Could you check a few things on this model? Use its own coordinates, in mm. Face numbers are marked on the shaded views. A direction names the side the tool comes from. Give positions to 0.01 mm unless a question says otherwise; leave off trailing zeros. Order: outer loops, then holes, each group sorted by start corner. A loop starts at its lowest first (then second) coordinate and runs counter-clockwise, first axis right, second up. Notation, with made-up numbers: (-27, 23) -> (-1, 23) arc R25 cw to (-1, 62) -> close; hole circle Ø4 at (4.25, -13). An arc over 180 degrees is marked (long way). One line per item, written item: value.
```python
from build123d import *

# Parameters (mm, degrees)
F0_W     = 76.2
F0_H     = 76.2
F1_DEPTH = 5.08
F2_W     = 69.85
F2_H     = 69.85
F3_DEPTH = 95.25
F4_W     = 3.81
F4_H     = 3.81
F5_DEPTH = 100.33
F6_W     = 21.172609
F6_H     = 16.548711
F7_DEPTH = 73.026


with BuildPart() as f1:
    # F0 (on Top) → F1 (new body)
    with BuildSketch(Plane.XY):
        Rectangle(F0_W, F0_H)
    extrude(amount=F1_DEPTH)

    # F2 (on face) → F3 (join)
    with BuildSketch(Plane.XY.offset(5.08)):
        Rectangle(F2_W, F2_H)
    extrude(amount=F3_DEPTH)

    # F4 (on Top) → F5 (join)
    with BuildSketch(Plane.XY):
        with Locations((34.925, -34.925)):
            Rectangle(F4_W, F4_H)
        with Locations((-34.925, -34.925)):
            Rectangle(F4_W, F4_H)
        with Locations((-34.925, 34.925)):
            Rectangle(F4_W, F4_H)
        with Locations((34.925, 34.925)):
            Rectangle(F4_W, F4_H)
    extrude(amount=F5_DEPTH)

    # F6 (on face) → F7 (cut, through all)
    with BuildSketch(Plane.XZ.offset(34.925)):
        with Locations((-2.19027, 65.586423)):
            Rectangle(F6_W, F6_H)
    extrude(amount=-F7_DEPTH, mode=Mode.SUBTRACT)


solid = f1.part
```
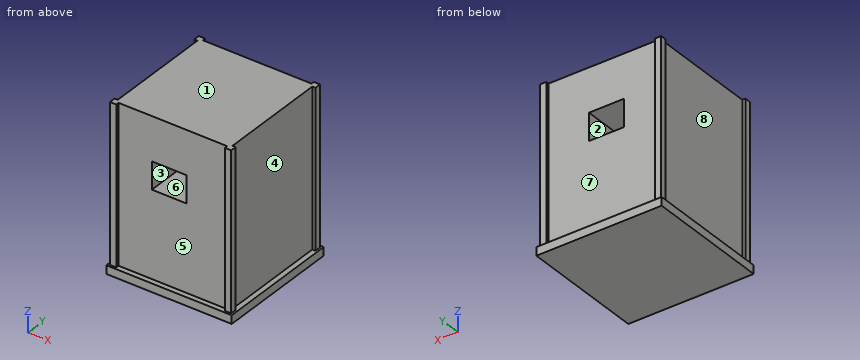
1) Suppose I cut it at A-A, the plane x = -9. Write out the boundary of the cut face in (y, z) (3 decimals), then the cut area to 3 significant figures.
Answer below:
outline: (-38.1, 0) -> (38.1, 0) -> (38.1, 5.08) -> (34.925, 5.08) -> (34.925, 57.312) -> (-34.925, 57.312) -> (-34.925, 5.08) -> (-38.1, 5.08) -> close; (-34.925, 73.861) -> (34.925, 73.861) -> (34.925, 100.33) -> (-34.925, 100.33) -> close
area: 5,880 mm2
2) For the marked faces 5, 6, 7 and 8, which set-ups out of +Z, -Z, +X, -X, +Y, -Y let a thin tool reach every point of the face, with its end or its side?
Answer below:
face 5: +Z, -Y
face 6: +Y, -Y
face 7: +Z, +Y
face 8: +Z, -X
3) Suppose I cut it at C-C, the plane x = 17. Write out the boundary of the cut face in (y, z) (3 decimals).
Answer below:
outline: (-38.1, 0) -> (38.1, 0) -> (38.1, 5.08) -> (34.925, 5.08) -> (34.925, 100.33) -> (-34.925, 100.33) -> (-34.925, 5.08) -> (-38.1, 5.08) -> close
4) Suppose I cut it at B-B, the plane y = -18. Write out the boundary of the cut face in (x, z) (3 decimals).
Answer below:
outline: (-38.1, 0) -> (38.1, 0) -> (38.1, 5.08) -> (34.925, 5.08) -> (34.925, 100.33) -> (-34.925, 100.33) -> (-34.925, 5.08) -> (-38.1, 5.08) -> close; hole (-12.777, 57.312) -> (8.396, 57.312) -> (8.396, 73.861) -> (-12.777, 73.861) -> close
5) For P1, Ø0.6, axis at y = -36, z = 62.5, coming from the -X side; P2, Ø6, axis at x = -19.5, z = 16, coming from the -Y side (3 decimals); P3, Ø1.5, axis at x = -36, z = 76, coming from the -Y side; P4, Ø5, axis at x = 1.5, y = 26, coming from the -Z side, each with a flat end and sliding along its axis, tell me the tip position at first contact or that it passes through.
Answer below:
P1: stops at x = -36.83
P2: stops at y = -34.925
P3: stops at y = -36.83
P4: stops at z = 0
6) We'd pull the mould along Z, two halves only. Please class the marked faces 1, 2, 3 and 4: +Z half, -Z half, draft (parallel to the pull), parting line (faces both ways), or undercut.
Answer below:
face 1: +Z half
face 2: undercut
face 3: undercut
face 4: draft
7) If I drill on line 1 along Z through (x, y) = (3.5, -16.5); line 2 along X through (y, z) = (16, 48) (3 decimals); line 3 along X through (y, z) = (10, 65) (3 decimals), over which ranges is the centre line in solid material (lowest first)?
Answer below:
line 1: z = 0 to 57.31, 73.86 to 100.33
line 2: x = -34.925 to 34.925
line 3: x = -34.925 to -12.777, 8.396 to 34.925
8) Suppose I cut it at D-D, the plane z = 22.5. Write out the boundary of the cut face in (x, y) (3 decimals).
Answer below:
outline: (-36.83, -36.83) -> (-33.02, -36.83) -> (-33.02, -34.925) -> (33.02, -34.925) -> (33.02, -36.83) -> (36.83, -36.83) -> (36.83, -33.02) -> (34.925, -33.02) -> (34.925, 33.02) -> (36.83, 33.02) -> (36.83, 36.83) -> (33.02, 36.83) -> (33.02, 34.925) -> (-33.02, 34.925) -> (-33.02, 36.83) -> (-36.83, 36.83) -> (-36.83, 33.02) -> (-34.925, 33.02) -> (-34.925, -33.02) -> (-36.83, -33.02) -> close
